```python
from build123d import *

# Parameters (mm, degrees)
SKETCH1_W               = 90
SKETCH1_H               = 7
SKETCH1_R               = 1.5
BOSS_EXTRUDE1_DEPTH     = 3.2
CUT_EXTRUDE1_DEPTH      = 91.328511556
CUT_EXTRUDE1_DEPTH_BACK = 91.328511556
FILLET1_R               = 1.5


with BuildPart() as part:
    # Sketch1 → Boss-Extrude1 (new body)
    with BuildSketch(Plane(origin=(0, 0, 0), x_dir=(1, 0, 0), z_dir=(0, 1, 0))):
        with Locations((45, 3.5)):
            Rectangle(SKETCH1_W, SKETCH1_H)
        with Locations(Location((5, 3.5, 0), (0, 0, 270))):
            Circle(SKETCH1_R, mode=Mode.SUBTRACT)
        with Locations(Location((85, 3.5, 0), (0, 0, 270))):
            Circle(SKETCH1_R, mode=Mode.SUBTRACT)
    extrude(amount=BOSS_EXTRUDE1_DEPTH)

    # Sketch2 → Cut-Extrude1 (cut, two sides: drawn at the far end of the back side and taken through both)
    with BuildSketch(Plane(origin=(90, 0, 0), x_dir=(0, 0, -1), z_dir=(1, 0, 0)).offset(-CUT_EXTRUDE1_DEPTH_BACK)):
        with BuildLine():
            Line((0, 0), (7, 0))
            ThreePointArc((7, 0), (3.5, 0.165912527), (0, 0))
        make_face()
    extrude(amount=CUT_EXTRUDE1_DEPTH + CUT_EXTRUDE1_DEPTH_BACK, mode=Mode.SUBTRACT)

    # Fillet1
    fillet1_edges = [part.edges().sort_by_distance(p)[0] for p in [
        (0, 1.6, -7),
        (90, 1.6, -7),
        (90, 1.6, 0),
        (0, 1.6, 0),
    ]]
    fillet(fillet1_edges, radius=FILLET1_R)


solid = part.part
```
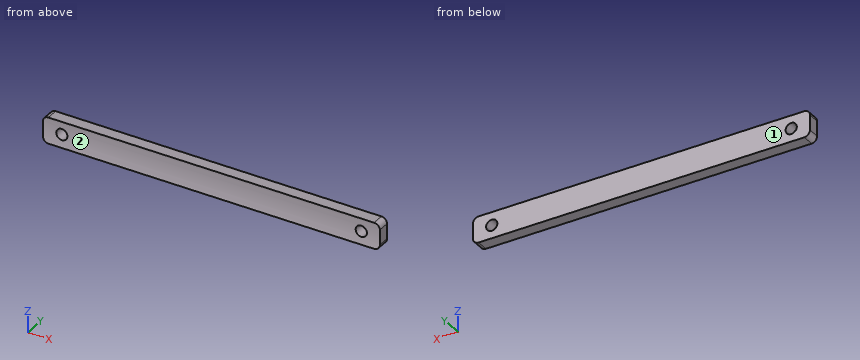
Work out the finished part from the listing and answer in its coordinate system (mm). Face numbers are marked on the shaded views. Coordinates: 2 decimals unless noted, no trailing zeros. Write each loop counter-clockwise with the first axis right and the second up, starting at its lowest first coordinate (ties: lowest second). Pieces come first, ordered by that corner, then holes. Notation, with made-up numbers: (87, -38.5) - (113, -38.5) arc R20 ccw to (113, -2.5) - close; hole circle Ø4 at (-20.75, -27.5). An arc over 180 degrees is marked (long way). Answer as a JSON object with one key per item and string values.
Q1. Find section D-D (x = 35.5). Write down the section's boundary in (y, z).
Results list:
{"outline": "(0, -7) - (3.2, -7) - (3.2, 0) - (0, 0) arc R37 cw to start"}
Q2. Given pin 1 Ø1.5 at (x, z) = (38, -6) entering from -Y; pin 2 Ø4 at (x, z) = (5, -3.5) entering from -Y, each flat-ended and moving along its own axis, determine where each tip first touches the part or whether it passes through.
Results list:
{"pin 1": "stops at y = 0.02", "pin 2": "stops at y = 0.11"}
Q3. Find section B-B (z = -3.5). Write down the section's boundary in (x, y).
Results list:
{"outline": "(0, 0.17) - (3.5, 0.17) - (3.5, 3.2) - (0, 3.2) - close; (6.5, 0.17) - (83.5, 0.17) - (83.5, 3.2) - (6.5, 3.2) - close; (86.5, 0.17) - (90, 0.17) - (90, 3.2) - (86.5, 3.2) - close"}
Q4. Consider L1, parallel to X at y = 1.35, z = -3.5; L2, parallel to X at y = 1.4, z = -2.75; L3, parallel to Z at x = 5, y = 1.45. Determine where each line is inside the solid, lowest interval first. Write a range as from..to.
Results list:
{"L1": "x = 0..3.5, 6.5..83.5, 86.5..90", "L2": "x = 0..3.7, 6.3..83.7, 86.3..90", "L3": "z = -7..-5, -2..0"}
Q5. For a pull along Z with two mould halves and no side action, classify the marked faces 1 and 2 as pulls with the +Z half, pulls with the -Z half, needs draft (parallel to the pull), parting line crosses it, or undercut.
Results list:
{"face 1": "needs draft", "face 2": "undercut"}
Q6. Find section A-A (x = 5). Write down the section's boundary in (y, z), plus the area to 3 significant figures.
Results list:
{"outline": "(0, -7) - (3.2, -7) - (3.2, -5) - (0.14, -5) arc R37 cw to start; (0, 0) arc R37 cw to (0.14, -2) - (3.2, -2) - (3.2, 0) - close", "area": "12.5 mm^2"}
Q7. Find section C-C (y = 1.95). Write down the section's boundary in (x, z).
Results list:
{"outline": "(0, -5.5) arc R1.5 ccw to (1.5, -7) - (88.5, -7) arc R1.5 ccw to (90, -5.5) - (90, -1.5) arc R1.5 ccw to (88.5, 0) - (1.5, 0) arc R1.5 ccw to (0, -1.5) - close; hole circle Ø3 at (5, -3.5); hole circle Ø3 at (85, -3.5)"}
